```python
from build123d import *

# Parameters (mm, degrees)
SKETCH1_W           = 139.7
SKETCH1_H           = 63.5
BOSS_EXTRUDE1_DEPTH = 9.525
SKETCH2_R           = 1.2192
SKETCH2_R_2         = 5.08
CUT_EXTRUDE1_DEPTH  = 9.525
SKETCH3_R           = 2.3368
CUT_EXTRUDE3_DEPTH  = 2.8448
SKETCH4_R           = 1.2192
CUT_EXTRUDE5_DEPTH  = 154.750010163


with BuildPart() as part:
    # Sketch1 → Boss-Extrude1 (new body)
    with BuildSketch(Plane(origin=(0, 0, 0), x_dir=(1, 0, 0), z_dir=(0, 1, 0))):
        with Locations((69.85, 31.75)):
            Rectangle(SKETCH1_W, SKETCH1_H)
    extrude(amount=BOSS_EXTRUDE1_DEPTH)

    # Sketch2 → Cut-Extrude1 (cut)
    with BuildSketch(Plane(origin=(0, 9.525, 0), x_dir=(1, 0, 0), z_dir=(0, 1, 0))):
        with Locations(Location((58.34888, 47.2567, 0), (0, 0, 270))):
            Circle(SKETCH2_R)
        with Locations(Location((89.36228, 47.2567, 0), (0, 0, 270))):
            Circle(SKETCH2_R)
        with Locations(Location((89.36228, 16.2433, 0), (0, 0, 270))):
            Circle(SKETCH2_R)
        with Locations(Location((58.34888, 16.2433, 0), (0, 0, 270))):
            Circle(SKETCH2_R)
        with Locations(Location((73.85558, 31.75, 0), (0, 0, 270))):
            Circle(SKETCH2_R_2)
    extrude(amount=-CUT_EXTRUDE1_DEPTH, mode=Mode.SUBTRACT)

    # Sketch3 → Cut-Extrude3 (cut)
    with BuildSketch(Plane.XZ.offset(-9.525)):
        with Locations(Location((6.35, -15.875, 0), (0, 0, 270))):
            Circle(SKETCH3_R)
        with Locations(Location((6.35, -31.75, 0), (0, 0, 270))):
            Circle(SKETCH3_R)
        with Locations(Location((6.35, -47.625, 0), (0, 0, 270))):
            Circle(SKETCH3_R)
        with Locations(Location((133.35, -47.625, 0), (0, 0, 270))):
            Circle(SKETCH3_R)
        with Locations(Location((133.35, -31.75, 0), (0, 0, 270))):
            Circle(SKETCH3_R)
        with Locations(Location((133.35, -15.875, 0), (0, 0, 270))):
            Circle(SKETCH3_R)
    extrude(amount=CUT_EXTRUDE3_DEPTH, mode=Mode.SUBTRACT)

    # Sketch4 → Cut-Extrude5 (cut, through all)
    with BuildSketch(Plane(origin=(0, 9.525, 0), x_dir=(1, 0, 0), z_dir=(0, 1, 0))):
        with Locations(Location((6.35, 47.625, 0), (0, 0, 270))):
            Circle(SKETCH4_R)
        with Locations(Location((6.35, 31.75, 0), (0, 0, 270))):
            Circle(SKETCH4_R)
        with Locations(Location((6.35, 15.875, 0), (0, 0, 270))):
            Circle(SKETCH4_R)
        with Locations(Location((133.35, 15.875, 0), (0, 0, 270))):
            Circle(SKETCH4_R)
        with Locations(Location((133.35, 31.75, 0), (0, 0, 270))):
            Circle(SKETCH4_R)
        with Locations(Location((133.35, 47.625, 0), (0, 0, 270))):
            Circle(SKETCH4_R)
    extrude(amount=-CUT_EXTRUDE5_DEPTH, mode=Mode.SUBTRACT)


solid = part.part
```
Design review of the part built by this model. Coordinates are the model's own, in mm. A direction names the side the tool comes from. Coordinates: 2 decimals unless noted, no trailing zeros. Answer as a JSON object with one key per item and string values.
Item 1: Machinability: for faces 1 (the cylindrical face through (135.32, 8.12, -48.88)), 2 (the cylindrical face through (59.558, 4.829, -47.415)), which of the approach directions +Z, -Z, +X, -X, +Y, -Y give a long, thin tool a straight path to every point of the face, cutting with its end or side? Answer none if there is none.
Outcome:
{"face 1": "+Y", "face 2": "+Y, -Y"}
Item 2: Wall thickness on probe 1 along Z at (x, y) = (133.35, 7.9); probe 2 along X at (y, z) = (1, -33.5); probe 3 along X at (y, z) = (3.5, -29): over which ranges is each line inside the solid? List them lowest first.
Outcome:
{"probe 1": "-63.5 to -49.96, -45.29 to -34.09, -29.41 to -18.21, -13.54 to 0", "probe 2": "0 to 69.09, 78.62 to 139.7", "probe 3": "0 to 69.58, 78.13 to 139.7"}
Item 3: Draft analysis for pull direction Z (two halves, no side actions). For faces 3 (the flat face through (69, 5, 0)), 4 (the flat face through (0, 5, -31)), 5 (the cylindrical face through (134.38, 3.39, -46.97)), 6 (the cylindrical face through (135.32, 8.12, -33.01)), state which applies: pulls with the +Z half, pulls with the -Z half, needs draft (parallel to the pull), parting line crosses it, or undercut.
Outcome:
{"face 3": "pulls with the +Z half", "face 4": "needs draft", "face 5": "undercut", "face 6": "undercut"}
Item 4: Insertion check: pin 1 Ø4 at (x, z) = (133.35, -47.625) entering from +Y. The pin has a flat end and moves straight along its axis. Give the tip position at first contact, or say it passes through.
Outcome:
{"pin 1": "y = 6.68"}
